Design review of the part shown in the three views and the two pictorial views. Dimensions are in mm from the part's minimum x, y and z. A direction names the side the tool comes from. Coordinates: 2 decimals unless noted, no trailing zeros. Loops run counter-clockwise (first coordinate to the right, second up) from the corner with the lowest first, then second, coordinate; pieces in that order, holes last. Notation, with made-up numbers: (67, 83) -> (74, 83) arc R31 cw to (74, 120) -> close; hole circle Ø8 at (14, 82.5). An arc over 180 degrees is marked (long way). Use a Markdown table: item, result. Add a question column.
Q1. Draft analysis for pull direction Z (two halves, no side actions). For the marked faces 3, 4, 5 and 6, state which applies: pulls with the +Z half, pulls with the -Z half, needs draft (parallel to the pull), parting line crosses it, or undercut.
Q2. For probe 1 along Y at (x, z) = (25, 5) (1 decimal); probe 2 along Y at (x, z) = (101.6, 5); probe 3 along Z at (x, y) = (25.4, 33), list the stretches that pass through material, from the lowest coordinate up.
Q3. Take a section at A-A on y = 12.7. Write out the cut boundary in (x, z) (1 decimal).
Q4. Take a section at D-D on x = 101.6. Write out the cut boundary in (y, z) (1 decimal), plus the area to 3 significant figures.
Q5. Take a section at B-B on x = 25.4. Write out the cut boundary in (y, z) (1 decimal).
Q6. Clearance check with flat-ended pins moving along their axes: pin 1 Ø11 at (x, y) = (101.6, 12.7) entering from +Z (3 decimals); pin 2 Ø1 at (y, z) = (23, 50) entering from -X; pin 3 Ø5 at (x, z) = (22.5, 53) entering from -Y; pin 4 Ø2 at (y, z) = (27.5, 49) entering from +X (1 decimal). State where each tip first meets the part, or that it passes through.
Q7. Take a section at C-C on z = 33. Write out the cut boundary in (x, y), plus the area to 3 significant figures.
Q8. For the marked faces 1 and 2, list the 3-axis set-ups (+Z, -Z, +X, -X, +Y, -Y) from which the entire face can be reached by the end or side of a thin tool; tool diameter is ignored.
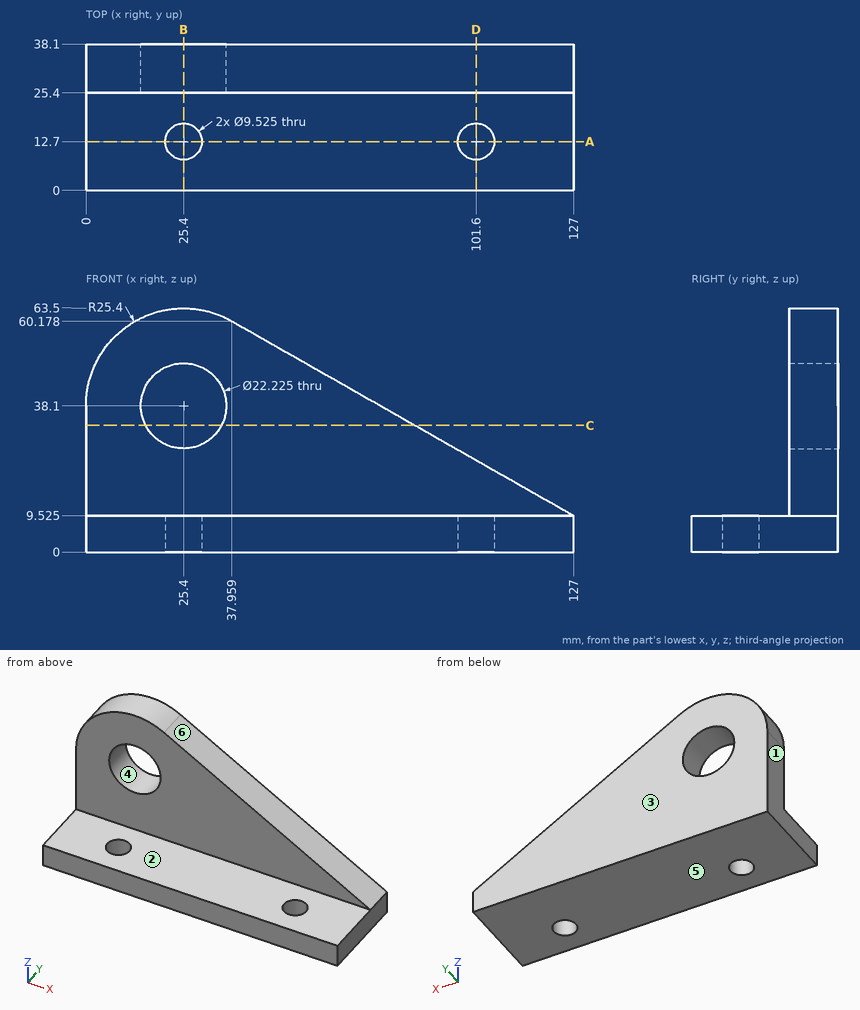
Answer list:
| question | item | result |
|---|---|---|
| 1 | face 3 | needs draft |
| 1 | face 4 | undercut |
| 1 | face 5 | pulls with the -Z half |
| 1 | face 6 | pulls with the +Z half |
| 2 | probe 1 | 0 to 8, 17.4 to 38.1 |
| 2 | probe 2 | 0 to 7.94, 17.46 to 38.1 |
| 2 | probe 3 | 0 to 26.99, 49.21 to 63.5 |
| 3 | outline | (0, 0) -> (20.6, 0) -> (20.6, 9.5) -> (0, 9.5) -> close; (30.2, 0) -> (96.8, 0) -> (96.8, 9.5) -> (30.2, 9.5) -> close; (106.4, 0) -> (127, 0) -> (127, 9.5) -> (106.4, 9.5) -> close |
| 4 | outline | (0, 0) -> (7.9, 0) -> (7.9, 9.5) -> (0, 9.5) -> close; (17.5, 0) -> (38.1, 0) -> (38.1, 24) -> (25.4, 24) -> (25.4, 9.5) -> (17.5, 9.5) -> close |
| 4 | area | 456 mm² |
| 5 | outline | (0, 0) -> (7.9, 0) -> (7.9, 9.5) -> (0, 9.5) -> close; (17.5, 0) -> (38.1, 0) -> (38.1, 27) -> (25.4, 27) -> (25.4, 9.5) -> (17.5, 9.5) -> close; (25.4, 49.2) -> (38.1, 49.2) -> (38.1, 63.5) -> (25.4, 63.5) -> close |
| 6 | pin 1 | z = 9.525 |
| 6 | pin 2 | through |
| 6 | pin 3 | y = 25.4 |
| 6 | pin 4 | x = 59.4 |
| 7 | outline | (0, 25.4) -> (15.53, 25.4) -> (15.53, 38.1) -> (0, 38.1) -> close; (35.27, 25.4) -> (85.73, 25.4) -> (85.73, 38.1) -> (35.27, 38.1) -> close |
| 7 | area | 838 mm² |
| 8 | face 1 | +Z, -Z, -X, +Y, -Y |
| 8 | face 2 | +Z, +X, -X, -Y |
